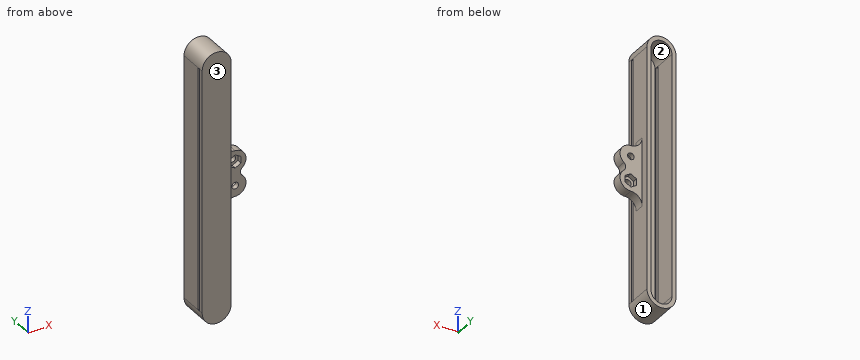
Autodesk Inventor part; units mm, degrees
ref_plane "Work Plane1" through (0, 6, 0) normal (0, -1, 0) x (1, 0, 0)
ref_plane "YZ Plane" through (0, 0, 0) normal (1, 0, 0) x (0, 1, 0)
ref_plane "XZ Plane" through (0, 0, 0) normal (0, 1, 0) x (-1, 0, 0)
sketch "Sketch1" plane through (0, 0, 0) normal (0, 1, 0) x (-1, 0, 0)
  line L0 (0, 0) -> (0, -130.5) construction
  line L1 (-5, -5) -> (-5, -125.5) construction
  line L2 (5, -125.5) -> (5, -5) construction
  arc A0 (5, -5) -> (-5, -5) centre (0, -5) ccw construction
  arc A1 (-5, -125.5) -> (5, -125.5) centre (0, -125.5) ccw construction
  line L3 (0, -65.25) -> (0, -71.25) construction
  line L4 (-5.2, -125.5) -> (-5.2, -5)
  arc A2 (5.2, -5) -> (-5.2, -5) centre (0, -5) ccw
  line L5 (5.2, -5) -> (5.2, -125.5)
  arc A3 (-5.2, -125.5) -> (5.2, -125.5) centre (0, -125.5) ccw
  line L6 (7.2, -125.5) -> (7.2, -5)
  arc A4 (7.2, -5) -> (-7.2, -5) centre (0, -5) ccw
  line L7 (-7.2, -5) -> (-7.2, -125.5)
  arc A5 (-7.2, -125.5) -> (7.2, -125.5) centre (0, -125.5) ccw
  line L8 (0, -71.25) -> (-12.85, -71.25) construction
  circle A6 centre (-12.85, -71.25) radius 1.65
  line L9 (-7.2, -76.6) -> (-12.85, -76.6)
  arc A7 (-12.85, -65.9) -> (-12.85, -76.6) centre (-12.85, -71.25) ccw
  line L10 (-12.85, -65.9) -> (-7.2, -65.9)
  line L11 (0, -65.25) -> (0, -59.25) construction
  line L12 (0, -59.25) -> (-7.2, -59.25) construction
  line L13 (-7.2, -59.25) -> (-12.85, -59.25) construction
  circle A8 centre (-12.85, -59.25) radius 1.65
  arc A9 (-12.85, -53.9) -> (-12.85, -64.6) centre (-12.85, -59.25) ccw
  line L14 (-12.85, -64.6) -> (-7.2, -64.6)
  line L15 (-12.85, -53.9) -> (-7.2, -53.9)
  arc A10 (-16.2998, -67.1608) -> (-16.2998, -63.3392) centre (-17.9119, -65.25) ccw
  arc A11 (-7.2, -82.25) -> (-12.85, -76.6) centre (-12.85, -82.25) ccw
  arc A12 (-12.85, -53.9) -> (-7.2, -48.25) centre (-12.85, -48.25) ccw
  point P0 (-11.2, -71.25)
  point P1 (-11.2, -59.25)
  point P2 (-11.2, -59.25)
  dimension "d15" = 3.3
  dimension "d20" = 3.3
  dimension "d0" = 130.5
  dimension "d1" = 10
  dimension "d2" = 6
  dimension "d6" = 0.2
  dimension "d7" = 2
  dimension "d14" = 3.7
  dimension "d16" = 4
  dimension "d17" = 6
  dimension "d18" = 3.7
  dimension "d19" = 4
  dimension "d24" = 2.5
extrude "Extrusion1" add sketch "Sketch1" along normal blind 1 contours L4 A2 L5 A3
extrude "Extrusion2" add sketch "Sketch1" along normal blind 15 contours A5 L7 A4 L6
ref_plane "Work Plane1" through (0, 6, 0) normal (0, -1, 0) x (1, 0, 0)
extrude "Extrusion4" add sketch "Sketch1" along normal blind 5 from surface at 6 contours A11 L9 L7 | L7 L15 A12 | L9 A7 L10 L7 | L7 L14 A9 L15 | L10 A7 A10 A9 L14 L7
sketch "Sketch2" plane through (7.2, 0, -5) normal (1, 0, 0) x (0, 0, -1)
  line L0 (0, 0) -> (0, 15)
  line L1 (120.5, 0) -> (120.5, 15)
  line L2 (0, 3.5) -> (120.5, 3.5)
  line L3 (120.5, 3.5) -> (120.5, 2)
  line L4 (120.5, 2) -> (0, 2)
  line L5 (0, 2) -> (0, 3.5)
  line L6 (0, 0) -> (120.5, 0)
  point P0 (-5, 0)
  point P1 (0, 2)
  dimension "d28" = 2
  dimension "d31" = 1.5
extrude "Extrusion5" cut sketch "Sketch2" against normal through all contours L0 L2 L1 L4
sketch "Sketch3" plane through (7.2, 6, -82.25) normal (0, -1, 0) x (1, 0, 0)
  circle A0 centre (5.65, 23) radius 1.65
  line L0 (5.65, 26.2909) -> (8.5, 24.6454)
  line L1 (8.5, 24.6454) -> (8.5, 21.3546)
  line L2 (8.5, 21.3546) -> (5.65, 19.7091)
  line L3 (5.65, 19.7091) -> (2.8, 21.3546)
  line L4 (2.8, 21.3546) -> (2.8, 24.6454)
  line L5 (2.8, 24.6454) -> (5.65, 26.2909)
  point P0 (-7.2, 82.25)
  dimension "d32" = 5.7
sketch "Sketch4" plane through (7.2, 11, -48.25) normal (0, 1, 0) x (1, 0, 0)
  circle A0 centre (5.65, 23) radius 1.65
  line L0 (8.5, 24.6454) -> (8.5, 21.3546)
  line L1 (8.5, 21.3546) -> (5.65, 19.7091)
  line L2 (5.65, 19.7091) -> (2.8, 21.3546)
  line L3 (2.8, 21.3546) -> (2.8, 24.6454)
  line L4 (2.8, 24.6454) -> (5.65, 26.2909)
  line L5 (5.65, 26.2909) -> (8.5, 24.6454)
  point P0 (-7.2, -48.25)
  dimension "d33" = 5.7
extrude "Extrusion6" cut sketch "Sketch4" against normal blind 2.5
extrude "Extrusion7" cut sketch "Sketch3" against normal blind 2.5
properties part number "wiper_linkage_magnet_holder" material "ABS Plastic"
Check sheet for the modelled part. Datum: model origin and axes. Units: mm. Face numbers are marked on the shaded views. Round coordinates to 2 decimals unless told otherwise and drop trailing zeros. Order: outer loops, then holes, each group sorted by start corner. A loop starts at its lowest first (then second) coordinate and runs counter-clockwise, first axis right, second up. Notation, with made-up numbers: M 29.5,74 L 81.5,74 A13 ccw 81.5,85 Z; hole C 87.5,19.25 d7. An arc over 180 degrees is marked long. Answer in a Markdown table with one row per item.
(1) Section check B-B on y = 13. Record the boundary of the cut face in (x, z).
Findings:
| item | result |
|---|---|
| outline | M -7.2,-125.5 A7.2 ccw 7.2,-125.5 L 7.2,-5 A7.2 ccw -7.2,-5 Z; hole M -5.2,-125.5 A5.2 ccw 5.2,-125.5 L 5.2,-5 A5.2 ccw -5.2,-5 Z |
(2) Gauge pin test, flat ends, axial feed: pin 1 (2.5 mm diameter, centred on x = 12.85, z = -71.25, fed in from +Y); pin 2 (6 mm diameter, centred on x = 5, y = 9.5, fed in from +Z); pin 3 (4 mm diameter, centred on x = 7, y = 5, fed in from +Z); pin 4 (1.6 mm diameter, centred on x = -6, y = 2.5, fed in from +Z). Record the tip position at first contact, or that the pin passes through.
Findings:
| item | result |
|---|---|
| pin 1 | passes through |
| pin 2 | stops at z = 1.92 |
| pin 3 | stops at z = 0.18 |
| pin 4 | stops at z = -0.02 |
(3) Material ranges on line 1 along X through (y, z) = (7.85, -71.25); line 2 along Z through (x, y) = (12.85, 7.35); line 3 along X through (y, z) = (9.5, -101), recorded low to high. Write a range as from..to.
Findings:
| item | result |
|---|---|
| line 1 | x = -7.2..-5.2, 5.2..11.2, 14.5..18.2 |
| line 2 | z = -76.6..-72.9, -69.6..-62.54, -55.96..-53.9 |
| line 3 | x = -7.2..-5.2, 5.2..7.2 |
(4) Section check A-A on z = -59.25. Record the boundary of the cut face in (x, y).
Findings:
| item | result |
|---|---|
| outline | M -7.2,0 L 7.2,0 L 7.2,2 L 5.2,2 L 5.2,1 L -5.2,1 L -5.2,2 L -7.2,2 Z; M -7.2,3.5 L -5.2,3.5 L -5.2,15 L -7.2,15 Z; M 5.2,3.5 L 7.2,3.5 L 7.2,6 L 10,6 L 10,8.5 L 11.2,8.5 L 11.2,11 L 7.2,11 L 7.2,15 L 5.2,15 Z; M 14.5,8.5 L 15.7,8.5 L 15.7,6 L 18.2,6 L 18.2,11 L 14.5,11 Z |
(5) Draft check along X on the marked faces 1, 2 and 3. Enter one of: +X half, -X half, draft (parallel to the pull), parting line (faces both ways), or undercut.
Findings:
| item | result |
|---|---|
| face 1 | parting line |
| face 2 | undercut |
| face 3 | draft |
(6) Section check D-D on x = 0. Record the boundary of the cut face in (y, z).
Findings:
| item | result |
|---|---|
| outline | M 0,-132.7 L 15,-132.7 L 15,-130.7 L 1,-130.7 L 1,0.2 L 15,0.2 L 15,2.2 L 0,2.2 Z |
(7) Section check C-C on z = -124. Record the boundary of the cut face in (x, y), plus the area to 3 significant figures.
Findings:
| item | result |
|---|---|
| outline | M -7.2,0 L 7.2,0 L 7.2,2 L 5.2,2 L 5.2,1 L -5.2,1 L -5.2,2 L -7.2,2 Z; M -7.2,3.5 L -5.2,3.5 L -5.2,15 L -7.2,15 Z; M 5.2,3.5 L 7.2,3.5 L 7.2,15 L 5.2,15 Z |
| area | 64.4 mm^2 |
